Could you check a few things on this model? Use its own coordinates, in mm. Face numbers are marked on the shaded views. A direction names the side the tool comes from. Give positions to 0.01 mm unless a question says otherwise; leave off trailing zeros. Order: outer loops, then holes, each group sorted by start corner. A loop starts at its lowest first (then second) coordinate and runs counter-clockwise, first axis right, second up. Notation, with made-up numbers: (67, -6) -> (115, -6) arc R7 ccw to (115, 3) -> close; hole circle Ø7 at (60.25, 66.25). An arc over 180 degrees is marked (long way). Answer as CSV lines item,"result". Start each with the question number.
(1) Will these pins go through, and if not, where does the flat tip stop? pin 1 Ø9 at (y, z) = (10, -1) entering from +X; pin 2 Ø5.5 at (x, z) = (10.5, 1) entering from +Y; pin 3 Ø1 at (y, z) = (4, 0) entering from +X.
(2) On a 3-axis mill with a long thin cutter (end or side, diameter ignored), from which of +Z, -Z, +X, -X, +Y, -Y can I reach the whole of each face in a straight line? I mean the marked faces 5 and 6. Say none if no direction works.
(3) I want a section at A-A (z = 0). Please give me the cut outline in (x, y).
(4) I need wall thicknesses on L1, parallel to Z at x = 10, y = 1.7; L2, parallel to X at y = 11.5, z = 4. Which ranges of each line are inside material? Lowest first, please.
(5) I want a section at C-C (x = 12.5). Please give me the cut outline in (y, z).
(6) I want a section at D-D (z = -6). Please give me the cut outline in (x, y).
(7) We'd pull the mould along Z, two halves only. Please class the marked faces 1, 2, 3 and 4: released by +Z, released by -Z, zero draft, split by the parting line, or undercut.
(8) I want a section at B-B (y = 7.25). Please give me the cut outline in (x, z).
Autodesk Inventor part; units mm, degrees
ref_plane "YZ Plane" through (0, 0, 0) normal (1, 0, 0) x (0, 1, 0)
ref_plane "XZ Plane" through (0, 0, 0) normal (0, 1, 0) x (-1, 0, 0)
ref_plane "XY Plane" through (0, 0, 0) normal (0, 0, 1) x (1, 0, 0)
sketch "Sketch1" plane through (0, 0, 0) normal (0, 0, 1) x (1, 0, 0)
  line L0 (0, 0) -> (20, 0)
  line L1 (20, 0) -> (20, 1)
  line L2 (20, 1) -> (1, 20)
  line L3 (1, 20) -> (0, 20)
  line L4 (0, 20) -> (0, 0)
  dimension "d0" = 135
  dimension "d1" = 20
  dimension "d2" = 20
  dimension "d3" = 1
extrude "Extrusion1" add sketch "Sketch1" along normal mid plane 20
sketch "Sketch2" plane through (0, 0, 10) normal (0, -1, 0) x (1, 0, 0)
  circle A0 centre (10, -10) radius 3.57
  point P0 (0, -10)
  dimension "d6" = 7.14
extrude "Extrusion2" cut sketch "Sketch2" against normal blind 3.5
sketch "Sketch3" plane through (10, 3.5, 0) normal (0, -1, 0) x (1, 0, 0)
  circle A0 centre (0, 0) radius 3.57
  circle A1 centre (0, 0) radius 5.5
  point P0 (-10, 0)
  dimension "d9" = 11
extrude "Extrusion3" cut sketch "Sketch3" against normal up to next contours A0 | A1
sketch "Sketch4" plane through (0, 0, 10) normal (-1, 0, 0) x (0, 0, 1)
  circle A0 centre (-10, 10) radius 3.57
  point P0 (-10, 0)
  dimension "d12" = 7.14
extrude "Extrusion4" cut sketch "Sketch4" against normal blind 3.5
sketch "Sketch5" plane through (3.5, 10, 0) normal (-1, 0, 0) x (0, 0, 1)
  circle A0 centre (0, 0) radius 3.57
  circle A1 centre (0, 0) radius 5.5
  point P0 (0, -10)
  dimension "d15" = 11
extrude "Extrusion5" cut sketch "Sketch5" against normal up to next contours A0 | A1
properties part number "Black Angle Corner Connector"
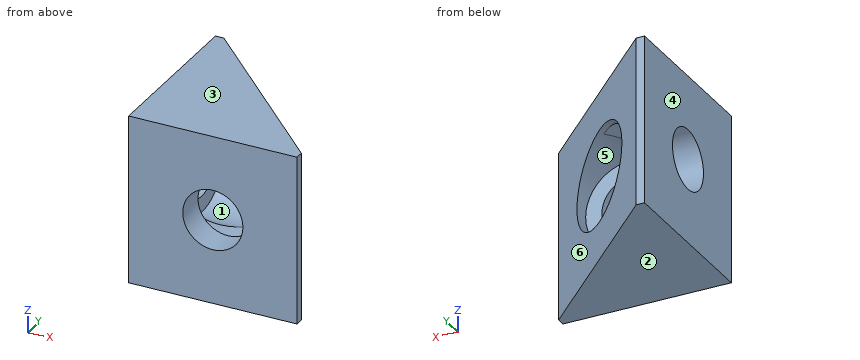
Final values:
1,pin 1,"x = 15.5"
1,pin 2,"y = 3.5"
1,pin 3,"x = 17.5"
2,face 5,"+Y"
2,face 6,"+Z, -Z, +X, +Y"
3,outline,"(0, 0) -> (6.43, 0) -> (6.43, 3.5) -> (4.5, 3.5) -> (4.5, 4.5) -> (3.5, 4.5) -> (3.5, 6.43) -> (0, 6.43) -> close; (0, 13.57) -> (3.5, 13.57) -> (3.5, 15.5) -> (4.5, 15.5) -> (4.5, 16.5) -> (1, 20) -> (0, 20) -> close; (13.57, 0) -> (20, 0) -> (20, 1) -> (15.5, 5.5) -> (15.5, 3.5) -> (13.57, 3.5) -> close"
4,L1,"-10 to -3.57, 3.57 to 10"
4,L2,"0 to 3.5"
5,outline,"(0, -10) -> (8.5, -10) -> (8.5, -4.9) -> (3.5, -4.9) -> (3.5, -2.55) -> (0, -2.55) -> close; (0, 2.55) -> (3.5, 2.55) -> (3.5, 4.9) -> (8.5, 4.9) -> (8.5, 10) -> (0, 10) -> close"
6,outline,"(0, 0) -> (20, 0) -> (20, 1) -> (1, 20) -> (0, 20) -> close"
7,face 1,"undercut"
7,face 2,"released by -Z"
7,face 3,"released by +Z"
7,face 4,"zero draft"
8,outline,"(0, -10) -> (13.75, -10) -> (13.75, -4.02) arc R5.5 cw to (7.25, -4.76) -> (3.5, -4.76) -> (3.5, -2.28) -> (0, -2.28) -> close; (0, 2.28) -> (3.5, 2.28) -> (3.5, 4.76) -> (7.25, 4.76) arc R5.5 cw to (13.75, 4.02) -> (13.75, 10) -> (0, 10) -> close"
